```python
from build123d import *

# Parameters (mm, degrees)
SKETCH1_W           = 23.85
SKETCH1_H           = 15.9
BOSS_EXTRUDE1_DEPTH = 3.1
SHELL1_T            = -1.2
SKETCH2_R           = 3.2
SKETCH2_R_2         = 2.4
BOSS_EXTRUDE2_DEPTH = 1.9
LPATTERN1_COUNT     = 2
LPATTERN1_PITCH     = 8


with BuildPart() as part:
    # Sketch1 → Boss-Extrude1 (new body)
    with BuildSketch(Plane(origin=(0, 0, 0), x_dir=(1, 0, 0), z_dir=(0, 1, 0))):
        Rectangle(SKETCH1_W, SKETCH1_H)
    extrude(amount=BOSS_EXTRUDE1_DEPTH)

    # Shell1
    shell1_openings = [part.faces().sort_by_distance(p)[0] for p in [
        (0, 0, 0),
    ]]
    offset(amount=SHELL1_T, openings=shell1_openings, kind=Kind.INTERSECTION)

    # Sketch2 → Boss-Extrude2 (add)
    with BuildSketch(Plane.XZ.offset(-1.9)):
        with Locations(Location((3.975, 0, 0), (0, 0, 270))):
            Circle(SKETCH2_R)
        with Locations(Location((3.975, 0, 0), (0, 0, 270))):
            Circle(SKETCH2_R_2, mode=Mode.SUBTRACT)
    boss_extrude2 = extrude(amount=BOSS_EXTRUDE2_DEPTH)

    # LPattern1: Boss-Extrude2 ×2
    with Locations(*[(-i * LPATTERN1_PITCH, 0, 0) for i in range(1, LPATTERN1_COUNT)]):
        add(boss_extrude2)


solid = part.part
```
The model under review builds one solid part; all positions refer to its coordinate system, in mm. A direction names the side the tool comes from. Round coordinates to 2 decimals unless told otherwise and drop trailing zeros. Loops run counter-clockwise (first coordinate to the right, second up) from the corner with the lowest first, then second, coordinate; pieces in that order, holes last. Notation, with made-up numbers: (5, -20) - (14, -20) arc R20 cw to (14, 18) - close; hole circle Ø6 at (40, -16). An arc over 180 degrees is marked (long way). Write each question's results on one line, items separated by ' | '. Start each with the question number.
Q1. Insertion check: P1, Ø2.5, axis at x = 3.5, z = 0, coming from the -Y side. The pin has a flat end and moves straight along its axis. Give the tip position at first contact, or say it passes through.
Q2. Draft analysis for pull direction Z (two halves, no side actions). For faces 3 (the flat face through (0, 2, 7.95)), 4 (the flat face through (0, 3.1, 0)), 5 (the cylindrical face through (7.148, 0.963, 0.417)), state which applies: pulls with the +Z half, pulls with the -Z half, needs draft (parallel to the pull), parting line crosses it, or undercut.
Q3. Take a section at D-D on x = -5. Give the boundary of the cut face in (y, z), plus the area to 3 significant figures.
Q4. Tool access review of faces 1 (the flat face through (-10.725, 1, 0)), 2 (the flat face through (0, 2, -7.95)): name each direction out of +Z, -Z, +X, -X, +Y, -Y from which nothing blocks a thin tool from reaching the whole face with its end or side.
Q5. Wall thickness on line 1 along X through (y, z) = (1.15, 0) (3 decimals); line 2 along Z through (x, y) = (8, 1.8); line 3 along X through (y, z) = (1.25, -5) (3 decimals): over which ranges is each line inside the solid? List them lowest first. Write a range as [from, to].
Q6. Take a section at B-B on x = -9. Give the boundary of the cut face in (y, z).
Q7. Take a section at A-A on z = 0. Give the boundary of the cut face in (x, y) (3 decimals), plus the area to 3 significant figures.
Q8. Take a section at C-C on z = 3.75. Give the boundary of the cut face in (x, y) (3 decimals), plus the area to 3 significant figures.
Data:
1) P1: stops at y = 1.9
2) face 3: pulls with the +Z half | face 4: needs draft | face 5: undercut
3) outline: (0, -7.95) - (3.1, -7.95) - (3.1, 7.95) - (0, 7.95) - (0, 6.75) - (1.9, 6.75) - (1.9, 3.05) - (0, 3.05) - (0, 2.19) - (1.9, 2.19) - (1.9, -2.19) - (0, -2.19) - (0, -3.05) - (1.9, -3.05) - (1.9, -6.75) - (0, -6.75) - close | area: 26.9 mm²
4) face 1: -Y | face 2: -Z, +X, -X, +Y, -Y
5) line 1: x = [-11.925, -10.725], [-7.225, -6.425], [-1.625, -0.825], [0.775, 1.575], [6.375, 7.175], [10.725, 11.925] | line 2: z = [-7.95, -6.75], [6.75, 7.95] | line 3: x = [-11.925, -10.725], [10.725, 11.925]
6) outline: (0, -7.95) - (3.1, -7.95) - (3.1, 7.95) - (0, 7.95) - (0, 6.75) - (1.9, 6.75) - (1.9, -6.75) - (0, -6.75) - close
7) outline: (-11.925, 0) - (-10.725, 0) - (-10.725, 1.9) - (-7.225, 1.9) - (-7.225, 0) - (-6.425, 0) - (-6.425, 1.9) - (-1.625, 1.9) - (-1.625, 0) - (-0.825, 0) - (-0.825, 1.9) - (0.775, 1.9) - (0.775, 0) - (1.575, 0) - (1.575, 1.9) - (6.375, 1.9) - (6.375, 0) - (7.175, 0) - (7.175, 1.9) - (10.725, 1.9) - (10.725, 0) - (11.925, 0) - (11.925, 3.1) - (-11.925, 3.1) - close | area: 39.3 mm²
8) outline: (-11.925, 0) - (-10.725, 0) - (-10.725, 1.9) - (10.725, 1.9) - (10.725, 0) - (11.925, 0) - (11.925, 3.1) - (-11.925, 3.1) - close | area: 33.2 mm²
